from build123d import *

# Parameters (mm, degrees)
SKETCH2_R           = 15
BOSS_EXTRUDE1_DEPTH = 20
SKETCH3_R           = 40.311288741
BOSS_EXTRUDE2_DEPTH = 50
FILLET1_R           = 50
FILLET2_R           = 50


with BuildPart() as part:
    # Sketch2 → Boss-Extrude1 (new, symmetric)
    with BuildSketch(Plane(origin=(0, 0, 0), x_dir=(1, 0, 0), z_dir=(0, 1, 0))):
        with BuildLine():
            Line((0, 35), (200, 35))
            Line((200, 35), (200, -35))
            Line((200, -35), (0, -35))
            ThreePointArc((0, -35), (-35, 0), (0, 35))
        make_face()
        with Locations(Location((0, 0, 0), (0, 0, 270))):
            Circle(SKETCH2_R, mode=Mode.SUBTRACT)
    extrude(amount=BOSS_EXTRUDE1_DEPTH, both=True)

    # Sketch3 → Boss-Extrude2 (add)
    with BuildSketch(Plane(origin=(200, 0, 0), x_dir=(0, 0, -1), z_dir=(1, 0, 0))):
        Circle(SKETCH3_R)
    extrude(amount=-BOSS_EXTRUDE2_DEPTH)

    # Fillet1
    # the kernel refuses this fillet: 50 mm, written as the material it adds along each edge
    with BuildSketch(Plane(origin=(150, -145, -35), x_dir=(-1, 0, 0), z_dir=(0, 1, 0))) as fillet1_piece_1_section:
        with BuildLine():
            CenterArc((FILLET1_R, -FILLET1_R), FILLET1_R, 90, 90)
            Line((0, -FILLET1_R), (0, 0))
            Line((0, 0), (FILLET1_R, 0))
        make_face()
    fillet1_piece_1 = extrude(amount=290, mode=Mode.PRIVATE)
    fillet1_piece_1 = fillet1_piece_1 & Plane(origin=(131.355668078, 0, 0), x_dir=(0, 0, -1), z_dir=(1, 0, 0)) * Cylinder(40.311288741, 781, mode=Mode.PRIVATE)
    add(fillet1_piece_1)
    with BuildSketch(Plane(origin=(150, 145, 35), x_dir=(0, 0, 1), z_dir=(0, -1, 0))) as fillet1_piece_2_section:
        with BuildLine():
            CenterArc((FILLET1_R, FILLET1_R), FILLET1_R, 180, 90)
            Line((0, FILLET1_R), (0, 0))
            Line((0, 0), (FILLET1_R, 0))
        make_face()
    fillet1_piece_2 = extrude(amount=290, mode=Mode.PRIVATE)
    fillet1_piece_2 = fillet1_piece_2 & Plane(origin=(131.35565772, 0, 0), x_dir=(0, 0, -1), z_dir=(1, 0, 0)) * Cylinder(40.311288741, 780, mode=Mode.PRIVATE)
    add(fillet1_piece_2)

    # Fillet2
    # the kernel refuses this fillet: 50 mm, written as the material it adds along each edge
    with BuildSketch(Plane(origin=(150, -20, -160), x_dir=(-1, 0, 0), z_dir=(0, 0, 1))) as fillet2_piece_1_section:
        with BuildLine():
            CenterArc((FILLET2_R, FILLET2_R), FILLET2_R, 180, 90)
            Line((0, FILLET2_R), (0, 0))
            Line((0, 0), (FILLET2_R, 0))
        make_face()
    fillet2_piece_1 = extrude(amount=320, mode=Mode.PRIVATE)
    fillet2_piece_1 = fillet2_piece_1 & Plane(origin=(135.236587788, 0, 0), x_dir=(0, 0, -1), z_dir=(1, 0, 0)) * Cylinder(40.311288741, 840, mode=Mode.PRIVATE)
    add(fillet2_piece_1)
    with BuildSketch(Plane(origin=(150, 20, -160), x_dir=(-1, 0, 0), z_dir=(0, 0, 1))) as fillet2_piece_2_section:
        with BuildLine():
            CenterArc((FILLET2_R, -FILLET2_R), FILLET2_R, 90, 90)
            Line((0, -FILLET2_R), (0, 0))
            Line((0, 0), (FILLET2_R, 0))
        make_face()
    fillet2_piece_2 = extrude(amount=320, mode=Mode.PRIVATE)
    fillet2_piece_2 = fillet2_piece_2 & Plane(origin=(135.236587787, 0, 0), x_dir=(0, 0, -1), z_dir=(1, 0, 0)) * Cylinder(40.311288741, 840, mode=Mode.PRIVATE)
    add(fillet2_piece_2)


solid = part.part
Work out the finished part from the listing and answer in its coordinate system (mm). A direction names the side the tool comes from. Give positions to 0.01 mm unless a question says otherwise; leave off trailing zeros. Loops run counter-clockwise (first coordinate to the right, second up) from the corner with the lowest first, then second, coordinate; pieces in that order, holes last. Notation, with made-up numbers: (-16, -26.5) -> (35, -26.5) arc R11 ccw to (35, -9.5) -> close; hole circle Ø10 at (48, 22). An arc over 180 degrees is marked (long way). Use a Markdown table: item, result. Add a question column.
1) Which of the six approach directions +Z, -Z, +X, -X, +Y, -Y give full straight-line access (tool end or side, diameter ignored) to faces 4 (the flat face through (51, 0, 35)), 5 (the flat face through (33, 20, 0)), 6 (the flat face through (49, 0, -35))?
2) The part is cut by section D-D, the plane z = 11. Determine the outline of the cut face in (x, y).
3) For a pull along Z with two mould halves and no side action, classify faces 1 (the cylindrical face through (0.66, -0.28, -14.985)), 2 (the cylindrical face through (108.834, 0.28, 35.787)), 3 (the cylindrical face through (161.811, 13.074, -38.132)) as +Z half, -Z half, draft (parallel to the pull), parting line (faces both ways), or undercut.
4) Consider line 1 along X through (y, z) = (8, 0); line 2 along Y through (x, z) = (-7.5, 22); line 3 along Z through (x, y) = (183, -1). Determine where each line is inside the solid, lowest interval first.
5) The part is cut by section A-A, the plane y = 0. Determine the outline of the cut face in (x, z).
6) The part is cut by section C-C, the plane x = 120. Determine the outline of the cut face in (y, z).
7) The part is cut by section B-B, the plane z = 0. Determine the outline of the cut face in (x, y), plus the area to 3 significant figures.
8) Each of these flat-tipped pins is pushed along its axis until it touches: P1, Ø4, axis at y = -1.5, z = 17, coming from the -X side; P2, Ø1.5, axis at x = 121, y = -8.5, coming from the +Z side; P3, Ø4, axis at y = -31, z = -7.5, coming from the -X side. Where does it stop, or does it pass through?
Reported:
| question | item | result |
|---|---|---|
| 1 | face 4 | +Z, -X, +Y, -Y |
| 1 | face 5 | +Z, -Z, -X, +Y |
| 1 | face 6 | -Z, -X, +Y, -Y |
| 2 | outline | (-33.23, -20) -> (-10.2, -20) -> (-10.2, 20) -> (-33.23, 20) -> close; (10.2, -20) -> (100, -20) arc R50 cw to (139.06, -38.78) -> (200, -38.78) -> (200, 38.78) -> (139.06, 38.78) arc R50 cw to (100, 20) -> (10.2, 20) -> close |
| 3 | face 1 | undercut |
| 3 | face 2 | +Z half |
| 3 | face 3 | parting line |
| 4 | line 1 | x = -35 to -15, 15 to 200 |
| 4 | line 2 | y = -20 to 20 |
| 4 | line 3 | z = -40.3 to 40.3 |
| 5 | outline | (0, -35) -> (100, -35) arc R50 cw to (122.43, -40.31) -> (200, -40.31) -> (200, 40.31) -> (122.43, 40.31) arc R50 cw to (100, 35) -> (0, 35) arc R35 ccw to start; hole circle Ø30 at (0, 0) |
| 6 | outline | (-24.17, -32.26) arc R40.31 ccw to (-9.51, -39.17) -> (9.51, -39.17) arc R40.31 ccw to (24.17, -32.26) -> (24.17, 32.26) arc R40.31 ccw to (9.51, 39.17) -> (-9.51, 39.17) arc R40.31 ccw to (-24.17, 32.26) -> close |
| 7 | outline | (-35, -20) -> (-15, -20) -> (-15, 20) -> (-35, 20) -> close; (15, -20) -> (100, -20) arc R50 cw to (140.23, -40.31) -> (200, -40.31) -> (200, 40.31) -> (140.23, 40.31) arc R50 cw to (100, 20) -> (15, 20) -> close |
| 7 | area | 11,100 mm^2 |
| 8 | P1 | stops at x = -31.62 |
| 8 | P2 | stops at z = 39.56 |
| 8 | P3 | stops at x = 128.62 |
